Design review of the part built by this model. Coordinates are the model's own, in mm. A direction names the side the tool comes from. Round coordinates to 2 decimals unless told otherwise and drop trailing zeros. Loops run counter-clockwise (first coordinate to the right, second up) from the corner with the lowest first, then second, coordinate; pieces in that order, holes last. Notation, with made-up numbers: M 80,17.25 L 130,17.25 A19 cw 130,39.25 Z; hole C 19.25,37 d2. An arc over 180 degrees is marked long. Use a Markdown table: item, result.
Autodesk Inventor part; units mm, degrees
ref_plane "YZ Plane" through (0, 0, 0) normal (1, 0, 0) x (0, 1, 0)
ref_plane "XZ Plane" through (0, 0, 0) normal (0, 1, 0) x (-1, 0, 0)
ref_plane "XY Plane" through (0, 0, 0) normal (0, 0, 1) x (1, 0, 0)
sketch "Sketch1" plane through (0, 0, 0) normal (0, 0, 1) x (1, 0, 0)
  line L0 (0, 0) -> (-7, 0) construction
  line L1 (-7, 0) -> (-7, 2.5)
  line L2 (-7, 2.5) -> (-6, 1.5)
  line L3 (-6, 1.5) -> (-6, 0)
  line L4 (-7, 2.5) -> (-11, 2.5)
  line L5 (-11, 2.5) -> (-11, 0)
  line L6 (-11, 0) -> (-7, 0)
  line L7 (-7, 0) -> (-7, 2.5)
  line L8 (-7, 0) -> (-6, 0)
  dimension "d0" = 7
  dimension "d1" = 45
  dimension "d2" = 1
  dimension "d3" = 2.5
  dimension "d5" = 11
extrude "Extrusion1" add sketch "Sketch1" along normal mid plane 24
mirror "Mirror1" about plane through (0, 0, 0) normal (1, 0, 0) of "Extrusion1"
sketch "Sketch2" plane through (-11, 0, 12) normal (0, -1, 0) x (1, 0, 0)
  line L0 (5, -24) -> (5, 0)
  line L1 (0, 0) -> (5, 0)
  line L2 (0, -24) -> (0, 0)
  line L3 (5, -24) -> (0, -24)
  line L4 (17, -24) -> (17, 0)
  line L5 (17, -24) -> (22, -24)
  line L6 (22, -24) -> (22, 0)
  line L7 (22, 0) -> (17, 0)
  line L8 (11, -12) -> (11, -11)
  line L9 (5, -24) -> (5, 0)
  arc A0 (4, -11) -> (18, -11) centre (11, -11) ccw
  line L10 (11, -12) -> (11, -13)
  arc A1 (4, -21.4853) -> (18, -21.4853) centre (11, -13) ccw
  line L11 (17, -24) -> (17, 0)
  line L12 (4, 0) -> (4, -24)
  line L13 (18, 0) -> (18, -24)
  line L14 (4, -11) -> (4, -21.4853)
  line L15 (18, -11) -> (18, -21.4853)
  dimension "d8" = 1
  dimension "d11" = 7
  dimension "d12" = 11
extrude "Extrusion2" add sketch "Sketch2" against normal up to surface (2.5 mm away) contours A1 L12 A0 L0 | L0 A0 L4 A1 | L4 A0 L13 A1
sketch "Sketch3" plane through (-11, 0, 12) normal (0, -1, 0) x (1, 0, 0)
  line L0 (5, -14.6056) -> (5, 0)
  line L1 (0, 0) -> (5, 0)
  line L2 (0, -24) -> (0, 0)
  line L3 (5, -24) -> (0, -24)
  line L4 (5, -24) -> (5, -22.2195)
  arc A0 (5, -22.2195) -> (17, -22.2195) centre (11, -13) ccw
  line L5 (17, -24) -> (17, -22.2195)
  line L6 (17, -24) -> (22, -24)
  line L7 (22, -24) -> (22, 0)
  line L8 (22, 0) -> (17, 0)
  line L9 (17, -14.6056) -> (17, 0)
  arc A1 (5, -14.6056) -> (17, -14.6056) centre (11, -11) ccw
  line L10 (5, -14.6056) -> (5, 0)
  arc A2 (5, -14.6056) -> (17, -14.6056) centre (11, -11) ccw
  line L11 (6, -6.101) -> (6, -2.3397)
  line L12 (16, -6.101) -> (16, -2.3397)
  arc A3 (17, -3) -> (16, -2.3397) centre (11, -11) ccw
  arc A4 (6, -2.3397) -> (5, -3) centre (11, -11) ccw
  arc A5 (17, -7.3944) -> (16, -6.101) centre (11, -11) ccw
  arc A6 (6, -6.101) -> (5, -7.3944) centre (11, -11) ccw
  line L13 (17, -3) -> (17, -7.3944)
  line L14 (17, -14.6056) -> (17, 0)
  line L15 (5, -3) -> (5, -7.3944)
  point P0 (11, -12)
  dimension "d15" = 1
  dimension "d16" = 1
  dimension "d17" = 10
extrude "Extrusion3" add sketch "Sketch3" against normal blind 1.5 contours L0 A4 L11 A6 | A5 L12 A3 L9
sketch "Sketch4" plane through (-11, 0, 12) normal (0, -1, 0) x (1, 0, 0)
  line L0 (5, -14.6056) -> (5, -7.3944) construction
  arc A0 (6, -6.101) -> (5, -7.3944) centre (11, -11) ccw construction
  line L1 (6, -6.101) -> (6, -2.3397) construction
  arc A1 (6, -2.3397) -> (5, -3) centre (11, -11) ccw construction
  line L2 (5, -3) -> (5, 0) construction
  line L3 (0, 0) -> (5, 0) construction
  line L4 (0, -24) -> (0, 0) construction
  line L5 (5, -24) -> (0, -24) construction
  line L6 (5, -24) -> (5, -22.2195) construction
  arc A2 (5, -22.2195) -> (17, -22.2195) centre (11, -13) ccw construction
  line L7 (17, -24) -> (17, -22.2195) construction
  line L8 (17, -24) -> (22, -24) construction
  line L9 (22, -24) -> (22, 0) construction
  line L10 (22, 0) -> (17, 0) construction
  line L11 (17, -3) -> (17, 0) construction
  arc A3 (17, -3) -> (16, -2.3397) centre (11, -11) ccw construction
  line L12 (16, -2.3397) -> (16, -6.101) construction
  arc A4 (17, -7.3944) -> (16, -6.101) centre (11, -11) ccw construction
  line L13 (17, -14.6056) -> (17, -7.3944) construction
  arc A5 (5, -14.6056) -> (17, -14.6056) centre (11, -11) ccw construction
  circle A6 centre (11, -13) radius 11
  circle A7 centre (11, -13) radius 19.3975
  point P0 (11, -12)
extrude "Extrusion4" cut sketch "Sketch4" against normal through all
chamfer "Chamfer1" distance 0.5 angle 45 2 edges at (-5, 0.75, 8.798) (5, 0.75, 8.798)
equation "\"d16\" = d15"
properties part number "bottom_clip" material "ABS Plastic"
1. Machinability: for faces 4 (the face through (6, 1, 1)), 5 (the face through (-5.5, 1.5, 7.1)), 6 (the face through (5, 1, 7)), which of the approach directions +Z, -Z, +X, -X, +Y, -Y give a long, thin tool a straight path to every point of the face, cutting with its end or side? Answer none if there is none.
Check values:
| item | result |
|---|---|
| face 4 | +Y, -Y |
| face 5 | +Z, +Y |
| face 6 | +Z, +Y, -Y |
2. Take a section at C-C on z = -1.5. Give the boundary of the cut face in (x, y).
Check values:
| item | result |
|---|---|
| outline | M -10.99,0 L -6,0 L -6,1.5 L -6.54,2.04 L -6.54,2.5 L -10.99,2.5 Z; M 6,0 L 10.99,0 L 10.99,2.5 L 6.54,2.5 L 6.54,2.04 L 6,1.5 Z |
3. Take a section at B-B on x = 0. Give the boundary of the cut face in (y, z).
Check values:
| item | result |
|---|---|
| outline | M 0,-12 L 2.5,-12 L 2.5,-6 L 0,-6 Z |
4. The part is to be moulded in two halves that separate along X. For faces 1 (the face through (11, 1, -1)), 2 (the face through (-11, 1, -1)), 3 (the face through (-5.53, 0.74, 5.29)), say which applies: pulls with the +X half, pulls with the -X half, needs draft (parallel to the pull), parting line crosses it, or undercut.
Check values:
| item | result |
|---|---|
| face 1 | pulls with the +X half |
| face 2 | pulls with the -X half |
| face 3 | undercut |
5. Take a section at A-A on z = -5.25. Give the boundary of the cut face in (x, y), and give its area (3 significant figures).
Check values:
| item | result |
|---|---|
| outline | M -10.15,0 L -3.15,0 L -3.15,2.5 L -10.15,2.5 Z; M 3.15,0 L 10.15,0 L 10.15,2.5 L 3.15,2.5 Z |
| area | 35.0 mm² |
6. Insertion check: pin 1 (0.8 mm diameter, centred on x = -5.5, z = 6, fed in from +Y); pin 2 (1.5 mm diameter, centred on x = 2, y = 1, fed in from +Z); pin 3 (0.8 mm diameter, centred on y = 0.5, z = 6.5, fed in from +X). Each pin has a flat end and moves straight along its axis. Give the tip position at first contact, or say it passes through.
Check values:
| item | result |
|---|---|
| pin 1 | stops at y = 1.5 |
| pin 2 | stops at z = -5.44 |
| pin 3 | stops at x = 8.4 |
7. Take a section at D-D on y = 2.25. Give the boundary of the cut face in (x, z).
Check values:
| item | result |
|---|---|
| outline | M -6.75,-0.85 L -6.75,7.69 A11 ccw long 6.75,7.69 L 6.75,-0.85 A7 cw Z |
8. Wall thickness on line 1 along Z through (x, y) = (6, 2); line 2 along Z through (x, y) = (-5.75, 1.1); line 3 along X through (y, z) = (1.3, -5): over which ranges is each line inside the solid? List them lowest first. Write a range as from..to.
Check values:
| item | result |
|---|---|
| line 1 | z = -10.22..-2.61 |
| line 2 | z = -10.38..-2.99, 4.99..8.38 |
| line 3 | x = -10.25..-3.61, 3.61..10.25 |
